from build123d import *

# Parameters (mm, degrees)
SKETCH1_R           = 9
SKETCH1_R_2         = 5.1
BOSS_EXTRUDE1_DEPTH = 16
SKETCH2_R           = 9
BOSS_EXTRUDE2_DEPTH = 12
SKETCH5_R           = 4.45
CUT_EXTRUDE1_DEPTH  = 8


with BuildPart() as part:
    # Sketch1 → Boss-Extrude1 (new body)
    with BuildSketch(Plane.XY):
        Circle(SKETCH1_R)
        Circle(SKETCH1_R_2, mode=Mode.SUBTRACT)
    extrude(amount=BOSS_EXTRUDE1_DEPTH)

    # Sketch2 → Boss-Extrude2 (add)
    with BuildSketch(Plane.XY.offset(16)):
        Circle(SKETCH2_R)
    extrude(amount=BOSS_EXTRUDE2_DEPTH)

    # Sketch5 → Cut-Extrude1 (cut)
    with BuildSketch(Plane.XY.offset(28)):
        Circle(SKETCH5_R)
    extrude(amount=-CUT_EXTRUDE1_DEPTH, mode=Mode.SUBTRACT)


solid = part.part
Part model, mm, in its own coordinate system. A direction names the side the tool comes from. Coordinates: 2 decimals unless noted, no trailing zeros. Order: outer loops, then holes, each group sorted by start corner. A loop starts at its lowest first (then second) coordinate and runs counter-clockwise, first axis right, second up. Notation, with made-up numbers: M 80,19 L 111,19 A14 cw 111,44 Z; hole C 74,-16 d4. An arc over 180 degrees is marked long. One line per question, with ' | ' between items.
Q1. Slice it at A-A (y = 0). Give the cut face in (x, z).
A:
outline: M -9,0 L -5.1,0 L -5.1,16 L 5.1,16 L 5.1,0 L 9,0 L 9,28 L 4.45,28 L 4.45,20 L -4.45,20 L -4.45,28 L -9,28 Z
Q2. Two-plate mould, pull along X, no slides. Class faces 1 (the face through (4, -4, 0)), 2 (the face through (-1.172, 8.923, 13.804)), 3 (the face through (-0.965, -4.344, 24.056)): +X half, -X half, draft (parallel to the pull), parting line (faces both ways), or undercut.
A:
face 1: draft | face 2: parting line | face 3: undercut
Q3. Slice it at C-C (z = 25.5). Give the cut face in (x, y), and give its area (3 significant figures).
A:
outline: C 0,0 d18; hole C 0,0 d8.9 | area: 192 mm^2
Q4. Slice it at D-D (z = 18.5). Give the cut face in (x, y).
A:
outline: C 0,0 d18
Q5. Pin check, flat tips, straight feed: P1, Ø2, axis at x = -2, y = 0, coming from the +Z side; P2, Ø8, axis at x = 6.5, z = 11.5, coming from the -Y side; P3, Ø1, axis at y = -5.5, z = 14.5, coming from the +X side. Stop position of each tip, or through.
A:
P1: stops at z = 20 | P2: stops at y = -8.65 | P3: stops at x = 7.48
Q6. 3-axis set-ups, long thin cutter, end or side, ignore diameter. For faces 4 (the face through (0, 0, 20)), 5 (the face through (2.4, -4.5, 7.9)), 6 (the face through (-4.1, 2.1, 28)): which of +Z, -Z, +X, -X, +Y, -Y reach the whole face in a straight line?
A:
face 4: +Z | face 5: -Z | face 6: +Z, +X, -X, +Y, -Y
Q7. Drill centre lines: line 1 (Y direction, x = 0, z = 25.5); line 2 (Y direction, x = 0, z = 9.25); line 3 (Z direction, x = -4.5, y = -1). Where is each one in solid material? Low to high.
A:
line 1: y = -9 to -4.45, 4.45 to 9 | line 2: y = -9 to -5.1, 5.1 to 9 | line 3: z = 16 to 28
